from build123d import *

# Parameters (mm, degrees)
SKETCH1_W           = 60
SKETCH1_H           = 47
BOSS_EXTRUDE1_DEPTH = 9.5
SKETCH1_3_R         = 1
BOSS_EXTRUDE2_DEPTH = 9
SKETCH1_4_R         = 2
BOSS_EXTRUDE3_DEPTH = 29.5
SKETCH1_5_R         = 19
BOSS_EXTRUDE4_DEPTH = 24
FILLET1_R           = 3
FILLET2_R           = 0.5


with BuildPart() as part:
    # Sketch1 → Boss-Extrude1 (new body)
    with BuildSketch(Plane(origin=(0, 0, 0), x_dir=(1, 0, 0), z_dir=(0, 1, 0))):
        Rectangle(SKETCH1_W, SKETCH1_H)
    extrude(amount=BOSS_EXTRUDE1_DEPTH)

    # Sketch1<3> → Boss-Extrude2 (add)
    with BuildSketch(Plane(origin=(0, 0, 0), x_dir=(1, 0, 0), z_dir=(0, 1, 0))):
        with Locations((-15.5, 16)):
            Circle(SKETCH1_3_R)
        with Locations((15.5, 16)):
            Circle(SKETCH1_3_R)
        with Locations((15.5, -16)):
            Circle(SKETCH1_3_R)
        with Locations((-15.5, -16)):
            Circle(SKETCH1_3_R)
    extrude(amount=-BOSS_EXTRUDE2_DEPTH)

    # Sketch1<4> → Boss-Extrude3 (add)
    with BuildSketch(Plane(origin=(0, 0, 0), x_dir=(1, 0, 0), z_dir=(0, 1, 0))):
        with Locations((13, 0)):
            Circle(SKETCH1_4_R)
        with Locations((-13, 0)):
            Circle(SKETCH1_4_R)
    extrude(amount=-BOSS_EXTRUDE3_DEPTH)

    # Sketch1<5> → Boss-Extrude4 (add)
    with BuildSketch(Plane(origin=(0, 0, 0), x_dir=(1, 0, 0), z_dir=(0, 1, 0))):
        Circle(SKETCH1_5_R)
    extrude(amount=-BOSS_EXTRUDE4_DEPTH)

    # Fillet1
    fillet1_edges = [part.edges().sort_by_distance(p)[0] for p in [
        (-30, 4.75, 23.5),
        (30, 4.75, 23.5),
        (30, 4.75, -23.5),
        (-30, 4.75, -23.5),
    ]]
    fillet(fillet1_edges, radius=FILLET1_R)

    # Fillet2
    fillet2_edges = [part.edges().sort_by_distance(p)[0] for p in [
        (0, 9.5, 23.5),
        (-30, 9.5, 0),
        (30, 9.5, 0),
        (0, 9.5, -23.5),
        (29.121320344, 9.5, -22.621320344),
        (-29.121320344, 9.5, -22.621320344),
        (29.121320344, 9.5, 22.621320344),
        (-29.121320344, 9.5, 22.621320344),
    ]]
    fillet(fillet2_edges, radius=FILLET2_R)


solid = part.part
Can you work these out from the model? Positions are in its coordinate system, mm. A direction names the side the tool comes from. Give positions to 0.01 mm unless a question says otherwise; leave off trailing zeros. Loops run counter-clockwise (first coordinate to the right, second up) from the corner with the lowest first, then second, coordinate; pieces in that order, holes last. Notation, with made-up numbers: (78, -24) -> (126, -24) arc R14 ccw to (126, -11) -> close; hole circle Ø5 at (-34, -14.5). An arc over 180 degrees is marked (long way). Use one line per item in the form item = value.
1) If we section it at B-B (x = 0): Please give me the cut outline in (y, z).
Answers:
outline = (-24, -19) -> (0, -19) -> (0, -23.5) -> (9, -23.5) arc R0.5 ccw to (9.5, -23) -> (9.5, 23) arc R0.5 ccw to (9, 23.5) -> (0, 23.5) -> (0, 19) -> (-24, 19) -> close
2) I need wall thicknesses on line 1 along Y through (x, z) = (-21, -11.5); line 2 along Y through (x, z) = (4, -2); line 3 along Z through (x, y) = (0.5, -12). Which ranges of each line are inside material? Lowest first, please.
Answers:
line_1 = 0 to 9.5
line_2 = -24 to 9.5
line_3 = -18.99 to 18.99
3) If we section it at A-A (y = -7): Please give me the cut outline in (x, z).
Answers:
outline = circle Ø38 at (0, 0); circle Ø2 at (-15.5, -16); circle Ø2 at (-15.5, 16); circle Ø2 at (15.5, -16); circle Ø2 at (15.5, 16)
4) We'd pull the mould along X, two halves only. Please class faces 5 (the face through (13, -29.5, 0)), 6 (the face through (-14.6, -26.7, 1.2)), 7 (the face through (-29.14, 4.56, 22.6)), 8 (the face through (15.96, -4.44, 16.89)): released by +X, released by -X, zero draft, split by the parting line, or undercut.
Answers:
face_5 = zero draft
face_6 = undercut
face_7 = released by -X
face_8 = undercut
5) Will these pins go through, and if not, where does the flat tip stop? pin 1 (6 mm diameter, centred on y = -3.5, z = -3, fed in from +X); pin 2 (12 mm diameter, centred on x = 6, z = -16.5, fed in from -Y); pin 3 (4 mm diameter, centred on x = 3.5, y = -18, fed in from +Z).
Answers:
pin_1 = 19
pin_2 = -24
pin_3 = 18.94
6) For faces 1 (the face through (-16, -9, 16)), 2 (the face through (-16, -9, -16)), 3 (the face through (15, -9, 16)), 4 (the face through (-15.04, -4.44, -15.11)), which set-ups out of +Z, -Z, +X, -X, +Y, -Y let a thin tool reach every point of the face, with its end or its side?
Answers:
face_1 = +Z, -X, -Y
face_2 = -Z, -X, -Y
face_3 = +Z, +X, -Y
face_4 = -Y
7) If we section it at C-C (z = 0): Please give me the cut outline in (x, y), plus the area to 3 significant figures.
Answers:
outline = (-30, 0) -> (-19, 0) -> (-19, -24) -> (-15, -24) -> (-15, -29.5) -> (-11, -29.5) -> (-11, -24) -> (11, -24) -> (11, -29.5) -> (15, -29.5) -> (15, -24) -> (19, -24) -> (19, 0) -> (30, 0) -> (30, 9) arc R0.5 ccw to (29.5, 9.5) -> (-29.5, 9.5) arc R0.5 ccw to (-30, 9) -> close
area = 1,530 mm²
8) If we section it at D-D (y = -18): Please give me the cut outline in (x, z).
Answers:
outline = circle Ø38 at (0, 0)
